Work out the finished part from the listing and answer in its coordinate system (mm). A direction names the side the tool comes from. Round coordinates to 2 decimals unless told otherwise and drop trailing zeros. Order: outer loops, then holes, each group sorted by start corner. A loop starts at its lowest first (then second) coordinate and runs counter-clockwise, first axis right, second up. Notation, with made-up numbers: (19, 35.25) - (26, 35.25) arc R16 cw to (26, 55.25) - close; hole circle Ø2 at (55, 16). An arc over 180 degrees is marked (long way). Use one line per item in the form item = value. Start each with the question number.
Q1. For a pull along X with two mould halves and no side action, classify faces 1 (the cylindrical face through (-19.52, -1.25, 25.49)), 2 (the cylindrical face through (3.05, -20.95, 22.77)), 3 (the flat face through (-25.561, -1, 23)) as +X half, -X half, draft (parallel to the pull), parting line (faces both ways), or undercut.
Q2. The part is cut by section A-A on x = 26. Determine the outline of the cut face in (y, z), plus the area to 3 significant figures.
Q3. The part is cut by section C-C on z = 21.75. Determine the outline of the cut face in (x, y), plus the area to 3 significant figures.
Q4. The part is cut by section B-B on y = -17.25. Determine the outline of the cut face in (x, z), plus the area to 3 significant figures.
Q5. Which of the six approach directions +Z, -Z, +X, -X, +Y, -Y give full straight-line access (tool end or side, diameter ignored) to faces 4 (the flat face through (3, -2, 32.654)), 5 (the flat face through (3, -2.794, 23)), 6 (the flat face through (-13, -2.54, 23)), 7 (the flat face through (5.554, -20.4, 19.2)), 8 (the flat face through (3, -2, 13.604))?
Q6. Find the intervals of material crossed by line 1 (Y direction, x = -9, z = 22); line 2 (X direction, y = -9, z = 32.75); line 3 (Z direction, x = 1, y = -1), in increasing order. Write a range as [from, to].
Q7. The part is cut by section D-D on z = 16. Determine the outline of the cut face in (x, y), plus the area to 3 significant figures.
Q8. Given P1, Ø4, axis at x = -13, z = 27, coming from the -Y side; P2, Ø6, axis at y = -18.5, z = 22, coming from the +X side; P3, Ø12, axis at x = -12.5, y = -7.5, coming from the +Z side, each flat-ended and moving along its own axis, determine where each tip first touches the part or whether it passes through.
from build123d import *

# Parameters (mm, degrees)
F0_W     = 57.15
F0_H     = 19.05
F0_R     = 2.38125
F1_DEPTH = 2.54
F2_W     = 5.08
F2_H     = 13.97
F3_DEPTH = 0.254
F5_DEPTH = 5.08


with BuildPart() as f1:
    # F0 (on Front) → F1 (new body)
    with BuildSketch(Plane.XZ):
        with Locations((3.013964, 23.129006)):
            Rectangle(F0_W, F0_H)
        with Locations((-19.211036, 23.129006)):
            Circle(F0_R, mode=Mode.SUBTRACT)
        with Locations((25.238964, 23.129006)):
            Circle(F0_R, mode=Mode.SUBTRACT)
    extrude(amount=F1_DEPTH)

    # F2 (on face) → F3 (join)
    with BuildSketch(Plane.XZ.offset(2.54)):
        with Locations((3.013964, 23.129006)):
            Rectangle(F2_W, F2_H)
    extrude(amount=F3_DEPTH)

    # F4 (on face) → F5 (join)
    with BuildSketch(Plane.YZ.offset(5.553964)):
        with BuildLine():
            Line((-2.54, 19.71271), (-2.54, 26.545301))
            ThreePointArc((-2.54, 26.545301), (-2.661883, 26.847016), (-2.794, 27.144391))
            Line((-2.794, 27.144391), (-2.794, 19.11362))
            ThreePointArc((-2.794, 19.11362), (-2.661883, 19.410996), (-2.54, 19.71271))
        make_face()
        with BuildLine():
            ThreePointArc((-2.794, 27.144391), (-2.661883, 26.847016), (-2.54, 26.545301))
            Line((-2.54, 26.545301), (-2.54, 32.654006))
            Line((-2.54, 32.654006), (-6.351263, 32.654006))
            ThreePointArc((-6.351263, 32.654006), (-22.226263, 23.129006), (-6.351263, 13.604006))
            Line((-6.351263, 13.604006), (-2.54, 13.604006))
            Line((-2.54, 13.604006), (-2.54, 19.71271))
            ThreePointArc((-2.54, 19.71271), (-2.661883, 19.410996), (-2.794, 19.11362))
            ThreePointArc((-2.794, 19.11362), (-20.956263, 23.129006), (-2.794, 27.144391))
        make_face()
    extrude(amount=-F5_DEPTH)


solid = f1.part
Found:
q1.face_1 = undercut
q1.face_2 = draft
q1.face_3 = -X half
q2.outline = (-2.54, 13.6) - (0, 13.6) - (0, 20.87) - (-2.54, 20.87) - close; (-2.54, 25.39) - (0, 25.39) - (0, 32.65) - (-2.54, 32.65) - close
q2.area = 36.9 mm²
q3.outline = (-25.56, -2.54) - (-21.15, -2.54) - (-21.15, 0) - (-25.56, 0) - close; (-17.27, -2.54) - (0.47, -2.54) - (0.47, -2.79) - (5.55, -2.79) - (5.55, -2.54) - (23.3, -2.54) - (23.3, 0) - (-17.27, 0) - close; (0.47, -22.14) - (5.55, -22.14) - (5.55, -20.86) - (0.47, -20.86) - close; (27.18, -2.54) - (31.59, -2.54) - (31.59, 0) - (27.18, 0) - close
q3.area = 133 mm²
q4.outline = (0.47, 14.04) - (5.55, 14.04) - (5.55, 15.59) - (0.47, 15.59) - close; (0.47, 30.67) - (5.55, 30.67) - (5.55, 32.22) - (0.47, 32.22) - close
q4.area = 15.8 mm²
q5.face_4 = +Z, +X, -X, +Y
q5.face_5 = +X, -X
q5.face_6 = +Z, -Z, -X, -Y
q5.face_7 = +Z, -Z, +X, -Y
q5.face_8 = -Z, +X, -X, +Y
q6.line_1 = [-2.54, 0]
q6.line_2 = [0.47, 5.55]
q6.line_3 = [13.6, 32.65]
q7.outline = (-25.56, -2.54) - (0.47, -2.54) - (0.47, -5.11) - (5.55, -5.11) - (5.55, -2.54) - (31.59, -2.54) - (31.59, 0) - (-25.56, 0) - close; (0.47, -19.54) - (5.55, -19.54) - (5.55, -17.75) - (0.47, -17.75) - close
q7.area = 167 mm²
q8.P1 = -2.54
q8.P2 = 5.55
q8.P3 = 32.65
